from build123d import *

# Parameters (mm, degrees)
F0_W          = 65.6000001021
F0_H          = 65.6000001021
F0_W_2        = 61.6
F0_H_2        = 61.6
F0_R          = 1.6
F1_DEPTH      = 2
F2_DEPTH      = 6
F3_W          = 7.3
F3_H          = 7.3
F4_DEPTH      = 2
F5_DEPTH      = 6.001
F6_W          = 19.25
F6_H          = 2.69
F7_DEPTH      = 2.001000051
F7_DEPTH_BACK = 63.601000051
F8_W          = 10.5
F8_H          = 2.69
F9_DEPTH      = 2.001000051
F11_DEPTH     = 3
F12_R         = 1.5
F13_DEPTH     = 8.001
F14_R         = 2


with BuildPart() as f1:
    # F0 (on Top) → F1 (new body)
    with BuildSketch(Plane.XY):
        with Locations((30.5, -30.5)):
            Rectangle(F0_W, F0_H)
        with Locations((30.5, -30.5)):
            Rectangle(F0_W_2, F0_H_2, mode=Mode.SUBTRACT)
        with Locations((30.5, -30.5)):
            Rectangle(F0_W_2, F0_H_2)
        with Locations((5, -56)):
            Circle(F0_R, mode=Mode.SUBTRACT)
        with Locations((56, -56)):
            Circle(F0_R, mode=Mode.SUBTRACT)
        with Locations((3.5, -3.5)):
            Circle(F0_R, mode=Mode.SUBTRACT)
        with Locations((57.5, -3.5)):
            Circle(F0_R, mode=Mode.SUBTRACT)
    extrude(amount=-F1_DEPTH)

    # F0 (on Top) → F2 (join)
    with BuildSketch(Plane.XY):
        with Locations((30.5, -30.5)):
            Rectangle(F0_W, F0_H)
        with Locations((30.5, -30.5)):
            Rectangle(F0_W_2, F0_H_2, mode=Mode.SUBTRACT)
    extrude(amount=F2_DEPTH)

    # F3 (on face) → F4 (join)
    with BuildSketch(Plane.XY):
        with Locations((57.65, -3.35)):
            Rectangle(F3_W, F3_H)
        with Locations((3.35, -3.35)):
            Rectangle(F3_W, F3_H)
        Polygon((7, -46), (-0.3, -46), (-0.3, -61.3), (15, -61.3), (15, -54), (7, -54), align=None)
        Polygon((61.3, -61.3), (61.3, -46), (54, -46), (54, -54), (46.3, -54), (46.3, -61.3), align=None)
    extrude(amount=F4_DEPTH)

    # F0 (on Top) → F5 (cut, through all)
    with BuildSketch(Plane.XY):
        with Locations((3.5, -3.5)):
            Circle(F0_R)
        with Locations((57.5, -3.5)):
            Circle(F0_R)
        with Locations((5, -56)):
            Circle(F0_R)
        with Locations((56, -56)):
            Circle(F0_R)
    extrude(amount=F5_DEPTH, mode=Mode.SUBTRACT)

    # F6 (on face) → F7 (cut, two sides)
    with BuildSketch(Plane(origin=(61.3, 0, 0), x_dir=(0, -1, 0), z_dir=(-1, 0, 0))) as f7_sk:
        with Locations((36.496, 4.655)):
            Rectangle(F6_W, F6_H)
    extrude(amount=-F7_DEPTH, mode=Mode.SUBTRACT)
    extrude(f7_sk.sketch, amount=F7_DEPTH_BACK, mode=Mode.SUBTRACT)

    # F8 (on face) → F9 (cut, through all)
    with BuildSketch(Plane.YZ.offset(-0.3)):
        with Locations((-17.588, 4.655)):
            Rectangle(F8_W, F8_H)
    extrude(amount=-F9_DEPTH, mode=Mode.SUBTRACT)

    # F10 (on face) → F11 (cut)
    with BuildSketch(Plane(origin=(0, 0, -2), x_dir=(1, 0, 0), z_dir=(0, 0, -1))):
        Polygon((1.9122867597, 6.25), (0.3245735195, 3.5), (1.9122867597, 0.75), (5.0877132403, 0.75), (6.6754264805, 3.5), (5.0877132403, 6.25), align=None)
        Polygon((55.9122867597, 0.75), (59.0877132403, 0.75), (60.6754264805, 3.5), (59.0877132403, 6.25), (55.9122867597, 6.25), (54.3245735195, 3.5), align=None)
        Polygon((6.5877132403, 53.25), (8.1754264805, 56), (6.5877132403, 58.75), (3.4122867597, 58.75), (1.8245735195, 56), (3.4122867597, 53.25), align=None)
        Polygon((54.4122867597, 53.25), (57.5877132403, 53.25), (59.1754264805, 56), (57.5877132403, 58.75), (54.4122867597, 58.75), (52.8245735195, 56), align=None)
    extrude(amount=-F11_DEPTH, mode=Mode.SUBTRACT)

    # F12 (on face) → F13 (cut, through all)
    with BuildSketch(Plane(origin=(0, 0, -2), x_dir=(1, 0, 0), z_dir=(0, 0, -1))):
        with Locations((30.5, 30.5)):
            Circle(F12_R)
        with Locations((30.5, 35.5)):
            Circle(F12_R)
        with Locations((26.1698729811, 33)):
            Circle(F12_R)
        with Locations((26.1698729811, 28)):
            Circle(F12_R)
        with Locations((30.5, 25.5)):
            Circle(F12_R)
        with Locations((34.8301270189, 28)):
            Circle(F12_R)
        with Locations((34.8301270189, 33)):
            Circle(F12_R)
        with Locations((26.1698729811, 38)):
            Circle(F12_R)
        with Locations((21.8397459622, 30.5)):
            Circle(F12_R)
        with Locations((26.1698729811, 23)):
            Circle(F12_R)
        with Locations((34.8301270189, 23)):
            Circle(F12_R)
        with Locations((39.1602540378, 30.5)):
            Circle(F12_R)
        with Locations((34.8301270189, 38)):
            Circle(F12_R)
    extrude(amount=-F13_DEPTH, mode=Mode.SUBTRACT)

    # F14
    f14_edges = [f1.edges().sort_by_distance(p)[0] for p in [
        (-2.3, -63.3, 2),
        (-2.3, 2.3, 2),
        (63.3, 2.3, 2),
        (63.3, -63.3, 2),
    ]]
    fillet(f14_edges, radius=F14_R)


solid = f1.part
CAD build for the part. Positions are in the model's coordinates, mm. A direction names the side the tool comes from. Round coordinates to 2 decimals unless told otherwise and drop trailing zeros. Order: outer loops, then holes, each group sorted by start corner. A loop starts at its lowest first (then second) coordinate and runs counter-clockwise, first axis right, second up. Notation, with made-up numbers: (59, 89.25) - (83, 89.25) arc R32 ccw to (83, 126.25) - close; hole circle Ø5 at (10.5, -32). An arc over 180 degrees is marked (long way). Return JSON: item names as keys, results as strings.
(1) Cut at B-B (x = 30.5). Give the cut face in (y, z), then the cut area to 3 significant figures.
Answer key:
{"outline": "(-63.3, -2) - (-37, -2) - (-37, 0) - (-61.3, 0) - (-61.3, 6) - (-63.3, 6) - close; (-34, -2) - (-32, -2) - (-32, 0) - (-34, 0) - close; (-29, -2) - (-27, -2) - (-27, 0) - (-29, 0) - close; (-24, -2) - (2.3, -2) - (2.3, 6) - (0.3, 6) - (0.3, 0) - (-24, 0) - close", "area": "137 mm^2"}
(2) Wall check: probe 1 along X at (y, z) = (-38, -0.6); probe 2 along X at (y, z) = (-56, 1.3); probe 3 along X at (y, z) = (-5, 2.25). Give the ranges that are in metal, low to high. Write a range as from..to.
Answer key:
{"probe 1": "x = -2.3..24.67, 27.67..33.33, 36.33..63.3", "probe 2": "x = -2.3..3.4, 6.6..15, 46.3..54.4, 57.6..63.3", "probe 3": "x = -2.3..-0.3, 61.3..63.3"}
(3) Pin check, flat tips, straight feed: pin 1 Ø10 at (x, y) = (12, -43.5) entering from +Z; pin 2 Ø0.6 at (x, z) = (62.5, 5) entering from -Y; pin 3 Ø3.5 at (x, y) = (58, -3) entering from +Z; pin 4 Ø1.6 at (x, y) = (3, -3) entering from -Z. Stop position of each tip, or through.
Answer key:
{"pin 1": "stops at z = 0", "pin 2": "stops at y = -63.09", "pin 3": "stops at z = 2", "pin 4": "passes through"}
(4) Cut at A-A (y = -25.5). Give the cut face in (x, z), then the cut area to 3 significant figures.
Answer key:
{"outline": "(-2.3, -2) - (29, -2) - (29, 0) - (-0.3, 0) - (-0.3, 6) - (-2.3, 6) - close; (32, -2) - (63.3, -2) - (63.3, 6) - (61.3, 6) - (61.3, 0) - (32, 0) - close", "area": "149 mm^2"}
(5) Pull direction X, two halves, no side cores. Call faces 5 (the face through (56, -58.75, -1)), 6 (the face through (62.73, -62.7, 2.06)), 7 (the face through (30, 2.3, 2)): +X half, -X half, draft (parallel to the pull), parting line (faces both ways), or undercut.
Answer key:
{"face 5": "undercut", "face 6": "+X half", "face 7": "draft"}
(6) Cut at D-D (x = 22.5). Give the cut face in (y, z).
Answer key:
{"outline": "(-63.3, -2) - (-31.85, -2) - (-31.85, 0) - (-61.3, 0) - (-61.3, 6) - (-63.3, 6) - close; (-29.15, -2) - (2.3, -2) - (2.3, 6) - (0.3, 6) - (0.3, 0) - (-29.15, 0) - close"}
(7) Cut at C-C (y = -38). Give the cut face in (x, z).
Answer key:
{"outline": "(-2.3, -2) - (24.67, -2) - (24.67, 0) - (-0.3, 0) - (-0.3, 3.31) - (-2.3, 3.31) - close; (27.67, -2) - (33.33, -2) - (33.33, 0) - (27.67, 0) - close; (36.33, -2) - (63.3, -2) - (63.3, 3.31) - (61.3, 3.31) - (61.3, 0) - (36.33, 0) - close"}
(8) Tool access for faces 1 (the face through (5.86, -54.65, 1.49)), 2 (the face through (-1, -26.871, 5)), 3 (the face through (53.63, -57.394, -0.521)), 4 (the face through (7, -55, 2)): list every direction of +Z, -Z, +X, -X, +Y, -Y with a clear straight run to the whole face (end or side of a thin tool).
Answer key:
{"face 1": "+Z, -Z", "face 2": "+Z, +X, -X", "face 3": "-Z", "face 4": "+Z"}
